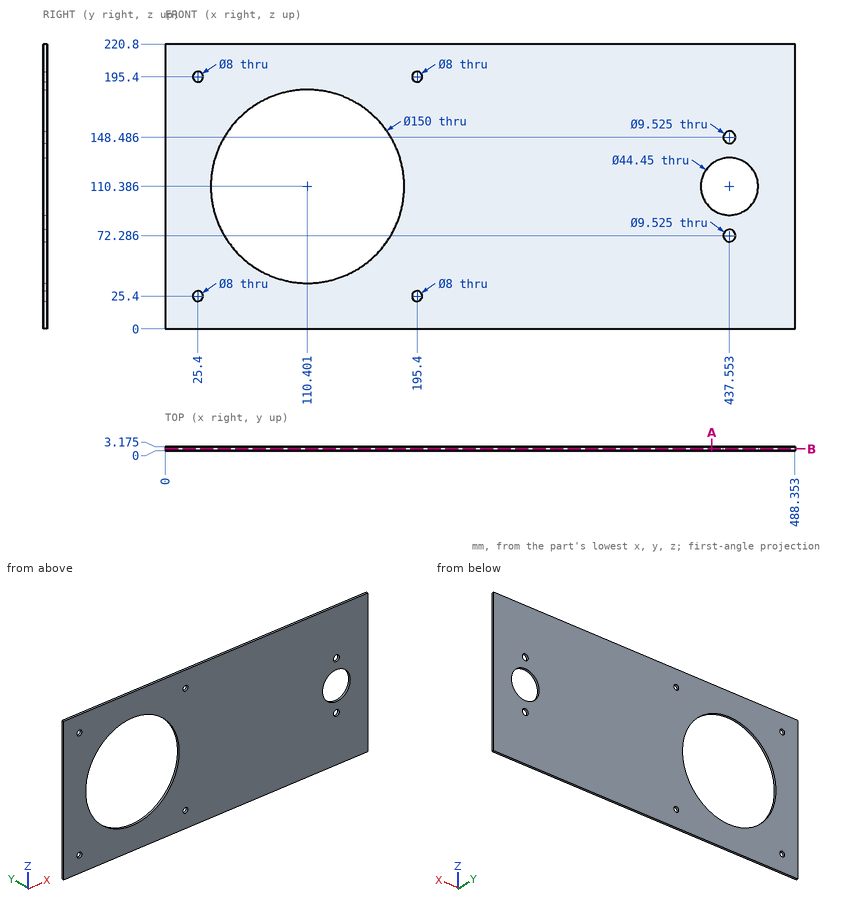
Here's the drawing with two shaded views (mm, measured from the low corner). I have some questions. Round coordinates to 2 decimals unless told otherwise and drop trailing zeros. Write each loop counter-clockwise with the first axis right and the second up, starting at its lowest first coordinate (ties: lowest second). Pieces come first, ordered by that corner, then holes. Notation, with made-up numbers: M 68.25,66.25 L 95.25,66.25 A11 cw 95.25,79.25 Z; hole C 19,41 d6. An arc over 180 degrees is marked long. Write each question's results on one line, items separated by ' | '. Start each with the question number.
1. Imagine slicing it at B-B on y = 1.65. Count the separate pieces of the cut face and the enclosed holes in it, and give its area (3 significant figures).
2. Imagine slicing it at A-A on x = 424. List the corners of the cut face in (y, z) for me (1 decimal).
3. I need wall thicknesses on L1, parallel to Z at x = 25.4, y = 1.65; L2, parallel to X at y = 2.55, z = 126 (1 decimal); L3, parallel to X at y = 2.05, z = 107.5. Which ranges of each line are inside material? Lowest first, please. Write a range as from..to.
Result sheet:
1) separate pieces: 1 | enclosed holes: 8 | area: 88,300 mm^2
2) outline: M 0,0 L 3.2,0 L 3.2,92.8 L 0,92.8 Z; M 0,128 L 3.2,128 L 3.2,220.8 L 0,220.8 Z
3) L1: z = 0..21.4, 29.4..191.4, 199.4..220.8 | L2: x = 0..37, 183.8..421.7, 453.4..488.4 | L3: x = 0..35.46, 185.35..415.52, 459.59..488.35
